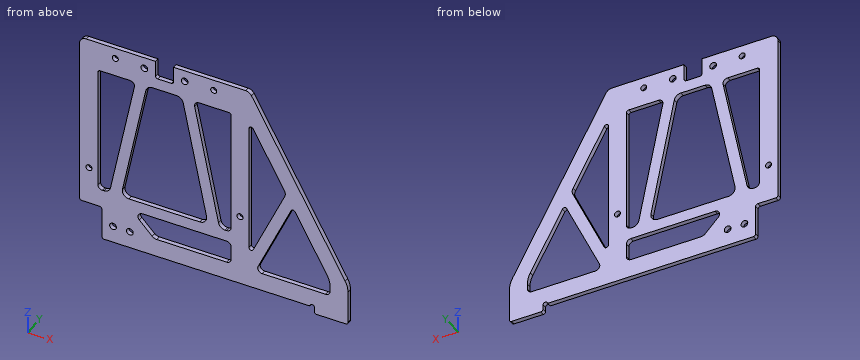
from build123d import *

# Parameters (mm, degrees)
SKETCH_1_R          = 1.5
EXTRUDE_1_DEPTH     = 2
SKETCH_4_R          = 1.35
SKETCH_4_R_2        = 1.5
SKETCH_4_W          = 8
SKETCH_4_H          = 8
CUT_EXTRUDE_2_DEPTH = 144.736738519
SKETCH_5_R          = 1
CUT_EXTRUDE_3_DEPTH = 144.736738519
FILLET_4_R          = 1
SKETCH_2_W          = 59.5
SKETCH_2_H          = 56.5
CUT_EXTRUDE_1_DEPTH = 144.736738519
EXTRUDE_1_2_DEPTH   = 2
FILLET_1_R          = 1
FILLET_3_R          = 3
FILLET_2_R          = 2
FILLET_5_R          = 10


with BuildPart() as part:
    # 草图1 → Extrude 1 (new body)
    with BuildSketch(Plane(origin=(0, 0, 0), x_dir=(1, 0, 0), z_dir=(0, 1, 0))):
        Polygon((0, 0), (95, 0), (95, 3), (110, 3), (110, -15), (66, -92.5), (-10, -92.5), (-10, -15), (0, -15), align=None)
        with Locations(Location((5, -7.5, 0), (0, 0, 270))):
            Circle(SKETCH_1_R, mode=Mode.SUBTRACT)
        with Locations(Location((12.5, -7.5, 0), (0, 0, 270))):
            Circle(SKETCH_1_R, mode=Mode.SUBTRACT)
    extrude(amount=EXTRUDE_1_DEPTH)

    # 草图4 → 切除-拉伸2 (cut, through all)
    with BuildSketch(Plane(origin=(0, 2, 0), x_dir=(1, 0, 0), z_dir=(0, 1, 0))):
        with Locations(Location((-5.75, -31.7, 0), (0, 0, 270))):
            Circle(SKETCH_4_R)
        with Locations(Location((6, -87.7, 0), (0, 0, 270))):
            Circle(SKETCH_4_R)
        with Locations(Location((50, -87.7, 0), (0, 0, 90))):
            Circle(SKETCH_4_R)
        with Locations(Location((61.75, -31.7, 0), (0, 0, 90))):
            Circle(SKETCH_4_R)
        with Locations(Location((19, -87.5, 0), (0, 0, 270))):
            Circle(SKETCH_4_R_2)
        with Locations(Location((37, -87.5, 0), (0, 0, 90))):
            Circle(SKETCH_4_R_2)
        with Locations((28, -88.5)):
            Rectangle(SKETCH_4_W, SKETCH_4_H)
    extrude(amount=-CUT_EXTRUDE_2_DEPTH, mode=Mode.SUBTRACT)

    # 草图5 → 切除-拉伸3 (cut, through all)
    with BuildSketch(Plane(origin=(0, 2, 0), x_dir=(1, 0, 0), z_dir=(0, 1, 0))):
        with Locations((94, 0)):
            Circle(SKETCH_5_R)
    extrude(amount=-CUT_EXTRUDE_3_DEPTH, mode=Mode.SUBTRACT)

    # 圆角4
    fillet_4_edges = [part.edges().sort_by_distance(p)[0] for p in [
        (95, 1, -3),
        (110, 1, -3),
    ]]
    fillet(fillet_4_edges, radius=FILLET_4_R)

    # 草图2 → 切除-拉伸1 (cut, through all)
    with BuildSketch(Plane(origin=(0, 2, 0), x_dir=(1, 0, 0), z_dir=(0, 1, 0))):
        with Locations((28, -51.25)):
            Rectangle(SKETCH_2_W, SKETCH_2_H)
        Polygon((65.75, -78.762270127), (102, -14.912838308), (102, -8), (65.75, -8), align=None)
        Polygon((23.313708499, -8), (57.75, -8), (57.75, -18), (13.313708499, -18), align=None)
    extrude(amount=-CUT_EXTRUDE_1_DEPTH, mode=Mode.SUBTRACT)

    # 草图3 → Extrude 1 2 (add)
    with BuildSketch(Plane(origin=(0, 2, 0), x_dir=(1, 0, 0), z_dir=(0, 1, 0))):
        Polygon((87.178028776, -48.003607703), (68.015439788, -6.942747632), (63.484560212, -9.057252368), (82.647149201, -50.118112438), align=None)
        Polygon((3.051710613, -21.505844915), (15.551710613, -82.005844915), (20.448289387, -80.994155085), (7.948289387, -20.494155085), align=None)
        Polygon((48.051710613, -20.494155085), (35.551710613, -80.994155085), (40.448289387, -82.005844915), (52.948289387, -21.505844915), align=None)
    extrude(amount=-EXTRUDE_1_2_DEPTH)

    # 圆角1
    fillet_1_edges = [part.edges().sort_by_distance(p)[0] for p in [
        (65.75, 1, 78.762270127),
        (-1.75, 1, 79.5),
        (57.75, 1, 79.5),
        (0, 1, 0),
        (65.75, 1, 13.911549779),
        (-10, 1, 15),
        (0, 1, 15),
        (85.389180361, 1, 44.17053199),
        (24, 1, 84.5),
        (32, 1, 84.5),
    ]]
    fillet(fillet_1_edges, radius=FILLET_1_R)

    # 圆角3
    fillet_3_edges = [part.edges().sort_by_distance(p)[0] for p in [
        (23.313708499, 1, 8),
        (66, 1, 92.5),
        (-10, 1, 92.5),
        (82.360819639, 1, 49.504576445),
        (20.139579659, 1, 79.5),
        (3.360420341, 1, 23),
        (8.46602594, 1, 23),
        (47.53397406, 1, 23),
        (52.639579659, 1, 23),
        (35.860420341, 1, 79.5),
    ]]
    fillet(fillet_3_edges, radius=FILLET_3_R)

    # 圆角2
    fillet_2_edges = [part.edges().sort_by_distance(p)[0] for p in [
        (102, 1, 8),
        (-1.75, 1, 23),
        (57.75, 1, 23),
        (13.313708499, 1, 18),
        (57.75, 1, 8),
        (57.75, 1, 18),
        (68.508846222, 1, 8),
        (15.03397406, 1, 79.5),
        (40.96602594, 1, 79.5),
    ]]
    fillet(fillet_2_edges, radius=FILLET_2_R)

    # 圆角5
    fillet_5_edges = [part.edges().sort_by_distance(p)[0] for p in [
        (102, 1, 14.912838308),
        (110, 1, 15),
    ]]
    fillet(fillet_5_edges, radius=FILLET_5_R)


solid = part.part
Could you check a few things on this model? Use its own coordinates, in mm. Coordinates: 2 decimals unless noted, no trailing zeros. Write each loop counter-clockwise with the first axis right and the second up, starting at its lowest first coordinate (ties: lowest second). Pieces come first, ordered by that corner, then holes. Notation, with made-up numbers: (10, 77) - (55, 77) arc R26 ccw to (55, 96) - close; hole circle Ø10 at (13.25, -38). An arc over 180 degrees is marked (long way). Write item = value, one per line.
1) Suppose I cut it at A-A on x = -5.75. Please give me the cut outline in (y, z), plus the area to 3 significant figures.
Result set:
outline = (0, 15) - (2, 15) - (2, 30.35) - (0, 30.35) - close; (0, 33.05) - (2, 33.05) - (2, 92.5) - (0, 92.5) - close
area = 150 mm2
2) Please list where these lines run through material, in increasing order: line 1 (X direction, y = 1.55, z = 7.5); line 2 (X direction, y = 0.7, z = 34); line 3 (X direction, y = 0.1, z = 22.5). Write a range as [from, to].
Result set:
line_1 = [0, 3.5], [6.5, 11], [14, 110]
line_2 = [-10, -1.75], [5.63, 10.74], [45.26, 50.37], [57.75, 65.75], [75.13, 80.64], [91.16, 99.21]
line_3 = [-10, 65.75], [69.76, 75.28], [97.69, 105.74]
3) Will these pins go through, and if not, where does the flat tip stop? pin 1 Ø0.6 at (x, y) = (-4.5, 1.5) entering from -Z; pin 2 Ø0.6 at (y, z) = (1, 11) entering from -X; pin 3 Ø6 at (x, z) = (70.5, 64) entering from -Y.
Result set:
pin_1 = 15
pin_2 = 0
pin_3 = through
4) Suppose I cut it at D-D on z = 39. Please give me the cut outline in (x, y), plus the area to 3 significant figures.
Result set:
outline = (-10, 0) - (-1.75, 0) - (-1.75, 2) - (-10, 2) - close; (6.67, 0) - (11.77, 0) - (11.77, 2) - (6.67, 2) - close; (44.23, 0) - (49.33, 0) - (49.33, 2) - (44.23, 2) - close; (57.75, 0) - (65.75, 0) - (65.75, 2) - (57.75, 2) - close; (77.46, 0) - (82.98, 0) - (82.98, 2) - (77.46, 2) - close; (88.32, 0) - (96.37, 0) - (96.37, 2) - (88.32, 2) - close
area = 80.1 mm2
5) Suppose I cut it at C-C on z = 56. Please give me the cut outline in (x, y), plus the area to 3 significant figures.
Result set:
outline = (-10, 0) - (-1.75, 0) - (-1.75, 2) - (-10, 2) - close; (10.18, 0) - (15.28, 0) - (15.28, 2) - (10.18, 2) - close; (40.72, 0) - (45.82, 0) - (45.82, 2) - (40.72, 2) - close; (57.75, 0) - (65.75, 0) - (65.75, 2) - (57.75, 2) - close; (78.67, 0) - (86.72, 0) - (86.72, 2) - (78.67, 2) - close
area = 69.0 mm2
6) Suppose I cut it at B-B on x = 26.5. Please give me the cut outline in (y, z), plus the area to 3 significant figures.
Result set:
outline = (0, 0) - (2, 0) - (2, 8) - (0, 8) - close; (0, 18) - (2, 18) - (2, 23) - (0, 23) - close; (0, 79.5) - (2, 79.5) - (2, 84.5) - (0, 84.5) - close
area = 36.0 mm2
